The figure shows three views and two pictorial views of one solid part (mm, origin at its lowest corner). Answer the questions. A direction names the side the tool comes from. Coordinates: 2 decimals unless noted, no trailing zeros. Write each loop counter-clockwise with the first axis right and the second up, starting at its lowest first coordinate (ties: lowest second). Pieces come first, ordered by that corner, then holes.
Item 1: Determine the mould class of the marked faces 3, 4 and 5 for opening direction X: released by +X, released by -X, zero draft, split by the parting line, or undercut.
Item 2: Section C-C (z = 9.75) is taken. Give the vertices of the cut face in (x, y), then the cut area to 3 significant figures.
Item 3: A tool of negligible diameter and unlimited length cuts with its end or side. For the marked faces 1 and 2, from which of +Z, -Z, +X, -X, +Y, -Y can it reach the whole face along a straight path? Write none if from no direction.
Item 4: Straight lines are drawn through the part: probe 1 along Y at (x, z) = (22.5, 5.25); probe 2 along Z at (x, y) = (36.5, 7); probe 3 along Y at (x, z) = (15, 2). For each, find the intervals that lie inside material, in ascending order.
Item 5: Section A-A (x = 22.5) is taken. Give the vertices of the cut face in (y, z).
Item 6: Each of these flat-tipped pins is pushed along its axis until it touches: P1, Ø2, axis at y = 40, z = 14, coming from the +X side; P2, Ø8, axis at y = 36, z = 15, coming from the +X side; P3, Ø8, axis at y = 22.5, z = 6, coming from the +X side; P4, Ø5, axis at x = 22, z = 11, coming from the -Y side. Where does it stop, or does it pass through?
Item 7: Section D-D (y = 9.5) is taken. Give the vertices of the cut face in (x, z), then the cut area to 3 significant figures.
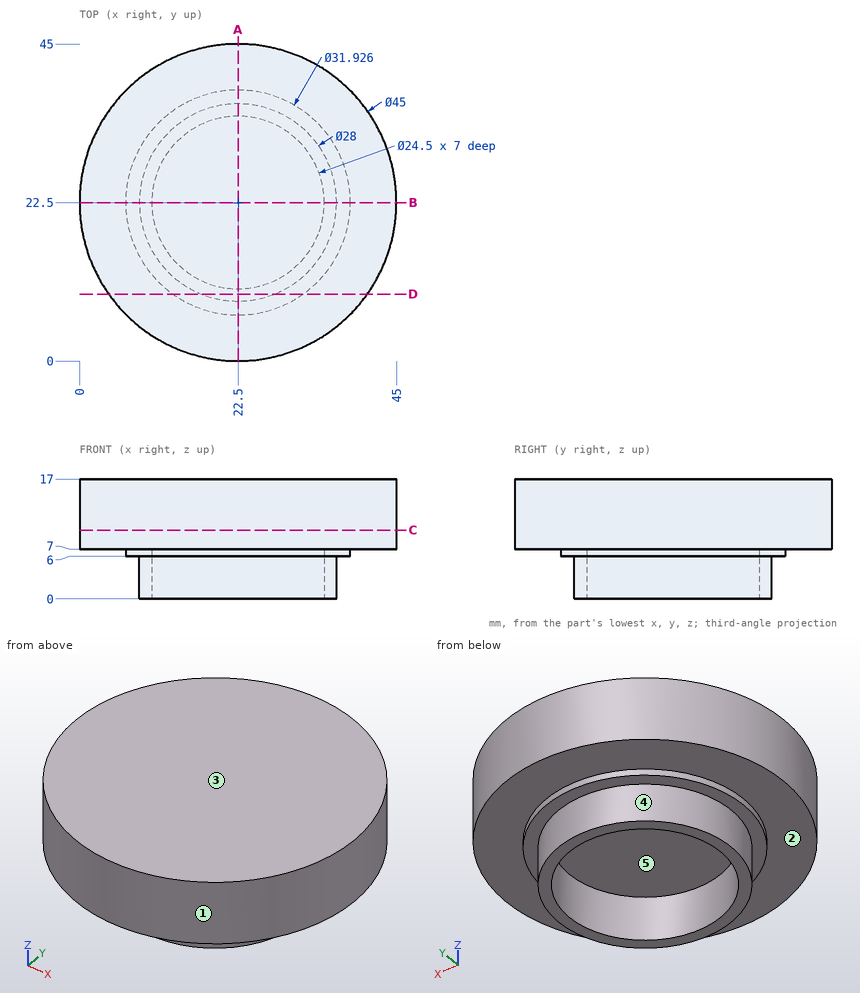
Established:
1. face 3: zero draft
1. face 4: split by the parting line
1. face 5: undercut
2. outline: circle Ø45 at (22.5, 22.5)
2. area: 1,590 mm2
3. face 1: +Z, -Z
3. face 2: -Z
4. probe 1: y = 8.5 to 10.25, 34.75 to 36.5
4. probe 2: z = 7 to 17
4. probe 3: y = 10.68 to 12.81, 32.19 to 34.32
5. outline: (0, 7) - (6.54, 7) - (6.54, 6) - (8.5, 6) - (8.5, 0) - (10.25, 0) - (10.25, 7) - (34.75, 7) - (34.75, 0) - (36.5, 0) - (36.5, 6) - (38.46, 6) - (38.46, 7) - (45, 7) - (45, 17) - (0, 17) - close
6. P1: stops at x = 37.8
6. P2: stops at x = 42.9
6. P3: stops at x = 45
6. P4: stops at y = 0
7. outline: (4.14, 7) - (13.24, 7) - (13.24, 6) - (17.3, 6) - (17.3, 0) - (27.7, 0) - (27.7, 6) - (31.76, 6) - (31.76, 7) - (40.86, 7) - (40.86, 17) - (4.14, 17) - close
7. area: 448 mm2
